Autodesk Inventor part; units mm, degrees
ref_plane "YZ Plane" through (0, 0, 0) normal (1, 0, 0) x (0, 1, 0)
ref_plane "XZ Plane" through (0, 0, 0) normal (0, 1, 0) x (-1, 0, 0)
ref_plane "XY Plane" through (0, 0, 0) normal (0, 0, 1) x (1, 0, 0)
sketch "Sketch1" plane through (0, 0, 0) normal (0, 1, 0) x (-1, 0, 0)
  line L0 (0, 0) -> (63, 0)
  line L1 (63, 0) -> (63, -7)
  line L2 (63, -7) -> (0, -7)
  line L3 (0, -7) -> (0, 0)
  circle A0 centre (31.5, -3) radius 1
  line L4 (31.5, 0) -> (31.5, -6) construction
  circle A1 centre (7, -3) radius 1
  circle A2 centre (56, -3) radius 1
  line L5 (63, -3) -> (0, -3) construction
  dimension "d0" = 63
  dimension "d1" = 7
  dimension "d2" = 2
  dimension "d3" = 31.5
  dimension "d5" = 7
  dimension "d6" = 2
  dimension "d9" = 3
extrude "Extrusion1" add sketch "Sketch1" along normal blind 2
equation "\"d3\" = 0.5 * d0"
equation "\"d6\" = d2"
properties part number "Seal"
Build history of the part. All positions in model axes, mm. Coordinates: 2 decimals unless noted, no trailing zeros. Order: outer loops, then holes, each group sorted by start corner. A loop starts at its lowest first (then second) coordinate and runs counter-clockwise, first axis right, second up.
Item 1: Saw through at A-A on x = -7. List the corners of the cut face in (y, z).
Filled in:
outline: (0, -7) - (2, -7) - (2, -4) - (0, -4) - close; (0, -2) - (2, -2) - (2, 0) - (0, 0) - close
Item 2: Mould opens along X. For faces 1 (the flat face through (-63, 1, -3)), 2 (the cylindrical face through (-6.263, 0.986, -3.676)), 3 (the flat face through (-31, 1, 0)) say: released by +X, released by -X, zero draft, split by the parting line, or undercut.
Filled in:
face 1: released by -X
face 2: undercut
face 3: zero draft
Item 3: Saw through at B-B on z = -3. List the corners of the cut face in (x, y).
Filled in:
outline: (-63, 0) - (-57, 0) - (-57, 2) - (-63, 2) - close; (-55, 0) - (-32.5, 0) - (-32.5, 2) - (-55, 2) - close; (-30.5, 0) - (-8, 0) - (-8, 2) - (-30.5, 2) - close; (-6, 0) - (0, 0) - (0, 2) - (-6, 2) - close
Item 4: Drill centre lines: L1, parallel to Z at x = -31.5, y = 1.05; L2, parallel to X at y = 0.9, z = -2.75. Where is each one in solid material? Low to high.
Filled in:
L1: z = -7 to -4, -2 to 0
L2: x = -63 to -56.97, -55.03 to -32.47, -30.53 to -7.97, -6.03 to 0
Item 5: Saw through at C-C on y = 0.75. List the corners of the cut face in (x, z), then the cut area to 3 significant figures.
Filled in:
outline: (-63, -7) - (0, -7) - (0, 0) - (-63, 0) - close; hole circle Ø2 at (-56, -3); hole circle Ø2 at (-31.5, -3); hole circle Ø2 at (-7, -3)
area: 432 mm2
